For this review, take the finished solid that the model builds, in its own axes (mm). A direction names the side the tool comes from. Give positions to 0.01 mm unless a question says otherwise; leave off trailing zeros. Order: outer loops, then holes, each group sorted by start corner. A loop starts at its lowest first (then second) coordinate and runs counter-clockwise, first axis right, second up. Notation, with made-up numbers: (-29.5, -18) - (-17.5, -18) arc R15 ccw to (-17.5, -10) - close; hole circle Ø6 at (-14.5, -32.75). An arc over 180 degrees is marked (long way). One line per item, written item: value.
```python
from build123d import *

# Parameters (mm, degrees)
F0_W     = 4
F0_H     = 10
F1_DEPTH = 8
F2_R     = 1.5
F3_DEPTH = 5
F5_DEPTH = 6
F7_D     = 1


with BuildPart() as f1:
    # F0 (on Right) → F1 (new body)
    with BuildSketch(Plane.YZ):
        Rectangle(F0_W, F0_H)
    extrude(amount=F1_DEPTH)

    # F2 (on face) → F3 (cut)
    with BuildSketch(Plane(origin=(0, 0, 0), x_dir=(0, -1, 0), z_dir=(-1, 0, 0))):
        with Locations((0, -3)):
            Circle(F2_R)
    extrude(amount=-F3_DEPTH, mode=Mode.SUBTRACT)

    # F4 (on face) → F5 (join)
    with BuildSketch(Plane.XY.offset(5)):
        with BuildLine():
            ThreePointArc((4, -2), (5.414214, -1.414214), (6, 0))
            ThreePointArc((6, 0), (5.414214, 1.414214), (4, 2))
            ThreePointArc((4, 2), (2, 0), (4, -2))
        make_face()
    extrude(amount=F5_DEPTH)

    # F7 (through all)
    with Locations(Plane.XY.offset(11)):
        with Locations((4, 0)):
            Hole(F7_D / 2)


solid = f1.part
```
(1) Draft analysis for pull direction X (two halves, no side actions). For faces 1 (the face through (3.5, 0.5, 11)), 2 (the face through (3.523, 0.15, -4.711)), 3 (the face through (4.4, -0.3, 4.6)), 4 (the face through (0, 0, 1)), state which applies: pulls with the +X half, pulls with the -X half, needs draft (parallel to the pull), parting line crosses it, or undercut.
Answers below:
face 1: needs draft
face 2: undercut
face 3: undercut
face 4: pulls with the -X half
(2) Take a section at B-B (z = -3). Write out the cut boundary in (x, y).
Answers below:
outline: (0, -2) - (8, -2) - (8, 2) - (0, 2) - (0, 1.5) - (5, 1.5) - (5, -1.5) - (0, -1.5) - close
(3) Take a section at C-C (x = 2.75). Write out the cut boundary in (y, z), then the cut area to 3 significant figures.
Answers below:
outline: (-2, -5) - (2, -5) - (2, 5) - (1.56, 5) - (1.56, 11) - (-1.56, 11) - (-1.56, 5) - (-2, 5) - close; hole circle Ø3 at (0, -3)
area: 51.7 mm^2
(4) Wall thickness on line 1 (X direction, y = 0, z = 5.5); line 2 (X direction, y = 0, z = -4.8); line 3 (Z direction, x = 2.5, y = 0.05): over which ranges is each line inside the solid? List them lowest first. Write a range as from..to.
Answers below:
line 1: x = 2..3.5, 4.5..6
line 2: x = 0..3.5, 4.5..8
line 3: z = -5..-4.5, -1.5..11
(5) Take a section at D-D (z = -0.25). Write out the cut boundary in (x, y), then the cut area to 3 significant figures.
Answers below:
outline: (0, -2) - (8, -2) - (8, 2) - (0, 2) - close; hole circle Ø1 at (4, 0)
area: 31.2 mm^2
(6) Machinability: for faces 5 (the face through (7, 0, 5)), 6 (the face through (2.46, -0.69, -4.33)), 7 (the face through (4, 2, 0)), which of the approach directions +Z, -Z, +X, -X, +Y, -Y give a long, thin tool a straight path to every point of the face, cutting with its end or side? Answer none if there is none.
Answers below:
face 5: +Z, +X
face 6: -X
face 7: +Z, -Z, +X, -X, +Y
(7) Take a section at A-A (y = 0.2). Write out the cut boundary in (x, z).
Answers below:
outline: (0, -5) - (3.54, -5) - (3.54, -4.49) - (0, -4.49) - close; (0, -1.51) - (3.54, -1.51) - (3.54, 11) - (2.01, 11) - (2.01, 5) - (0, 5) - close; (4.46, -5) - (8, -5) - (8, 5) - (5.99, 5) - (5.99, 11) - (4.46, 11) - (4.46, -1.51) - (5, -1.51) - (5, -4.49) - (4.46, -4.49) - close
